Here's how the part is built. I have some questions about the finished solid (model axes, mm). Coordinates: 2 decimals unless noted, no trailing zeros.
from build123d import *

# Parameters (mm, degrees)
SKETCH1_R           = 1.55
BOSS_EXTRUDE1_DEPTH = 7


with BuildPart() as part:
    # Sketch1 → Boss-Extrude1 (new body)
    with BuildSketch(Plane(origin=(0, 0, 0), x_dir=(1, 0, 0), z_dir=(0, 1, 0))):
        with BuildLine():
            Line((-94.441213517, -25.59472558), (-43.441213517, -25.59472558))
            Line((-43.441213517, -25.59472558), (-43.441213517, 22.40527442))
            Line((-43.441213517, 22.40527442), (-91.441213517, 22.40527442))
            ThreePointArc((-91.441213517, 22.40527442), (-93.562533861, 21.526594764), (-94.441213517, 19.40527442))
            Line((-94.441213517, 19.40527442), (-94.441213517, -25.59472558))
        make_face()
        with Locations(Location((-46.441213517, 19.40527442, 0), (0, 0, 270))):
            Circle(SKETCH1_R, mode=Mode.SUBTRACT)
        with Locations(Location((-46.441213517, -22.59472558, 0), (0, 0, 270))):
            Circle(SKETCH1_R, mode=Mode.SUBTRACT)
        with Locations(Location((-91.441213517, -22.59472558, 0), (0, 0, 270))):
            Circle(SKETCH1_R, mode=Mode.SUBTRACT)
        with Locations(Location((-91.441213517, 19.40527442, 0), (0, 0, 270))):
            Circle(SKETCH1_R, mode=Mode.SUBTRACT)
    extrude(amount=BOSS_EXTRUDE1_DEPTH)


solid = part.part
Q1. Please list where these lines run through material, in increasing order: probe 1 along Z at (x, y) = (-90.5, 0.5); probe 2 along Z at (x, y) = (-92, 0.75); probe 3 along X at (y, z) = (4, 23).
Q2. We'd pull the mould along Z, two halves only. Please class faces 1 (the flat face through (-67, 3, -22.405)), 2 (the flat face through (-69, 7, 1)), 3 (the cylindrical face through (-89.904, 3.451, -19.607)): pulls with the +Z half, pulls with the -Z half, needs draft (parallel to the pull), parting line crosses it, or undercut.
Q3. Will this pin go through, and if not, where does the flat tip stop? P1, Ø3, axis at x = -91.44, z = 22.59, coming from the -Y side.
Check values:
1. probe 1: z = -22.41 to -20.64, -18.17 to 21.36, 23.83 to 25.59
1. probe 2: z = -22.35 to -20.85, -17.96 to 21.15, 24.04 to 25.59
1. probe 3: x = -94.44 to -92.94, -89.95 to -47.94, -44.95 to -43.44
2. face 1: pulls with the -Z half
2. face 2: needs draft
2. face 3: undercut
3. P1: passes through
